from build123d import *

# Parameters (mm, degrees)
SKETCH_W     = 136
SKETCH_H     = 16
SKETCH_R     = 1.65
PAD_DEPTH    = 1
SKETCH001_W  = 106
SKETCH001_H  = 16
PAD001_DEPTH = 3
FILLET_R     = 2


with BuildPart() as part:
    # Sketch → Pad (new body)
    with BuildSketch(Plane.XY):
        Rectangle(SKETCH_W, SKETCH_H)
        with Locations((-60, 4)):
            Circle(SKETCH_R, mode=Mode.SUBTRACT)
        with Locations((-60, -4)):
            Circle(SKETCH_R, mode=Mode.SUBTRACT)
        with Locations((60, 4)):
            Circle(SKETCH_R, mode=Mode.SUBTRACT)
        with Locations((60, -4)):
            Circle(SKETCH_R, mode=Mode.SUBTRACT)
    extrude(amount=PAD_DEPTH)

    # Sketch001 → Pad001 (join)
    with BuildSketch(Plane.XY):
        Rectangle(SKETCH001_W, SKETCH001_H)
    extrude(amount=-PAD001_DEPTH)

    # Fillet
    fillet_edges = [part.edges().sort_by_distance(p)[0] for p in [
        (53, 8, -1.5),
        (53, -8, -1.5),
        (-53, -8, -1.5),
        (-53, 8, -1.5),
        (-68, 8, 0.5),
        (-68, -8, 0.5),
        (68, -8, 0.5),
        (68, 8, 0.5),
    ]]
    fillet(fillet_edges, radius=FILLET_R)


solid = part.part
The model under review builds one solid part; all positions refer to its coordinate system, in mm. A direction names the side the tool comes from. Give positions to 0.01 mm unless a question says otherwise; leave off trailing zeros. Order: outer loops, then holes, each group sorted by start corner. A loop starts at its lowest first (then second) coordinate and runs counter-clockwise, first axis right, second up. Notation, with made-up numbers: M 71,3 L 115,3 A34 cw 115,41 Z; hole C 70,-19 d2. An arc over 180 degrees is marked long. Answer in a Markdown table with one row per item. Add a question column.
1. Machinability: for faces 4 (the flat face through (53, 0, -1)), 5 (the cylindrical face through (-61.65, -3.93, 0.49)), which of the approach directions +Z, -Z, +X, -X, +Y, -Y give a long, thin tool a straight path to every point of the face, cutting with its end or side? Answer none if there is none.
2. To check wall thickness, follow line 1 along Y through (x, z) = (60, 0.85); line 2 along Z through (x, y) = (60.5, -1.5); line 3 along X through (y, z) = (-3, -1.7). State the ranges of each line that lie inside material, in increasing order.
3. Add section A-A on x = 60. State the section outline as (y, z) points.
4. Add section C-C on z = -2.2. State the section outline as (x, y) points, plus the area to 3 significant figures.
5. Add section D-D on y = 1.25. State the section outline as (x, z) points, plus the area to 3 significant figures.
6. Add section B-B on y = -4. State the section outline as (x, z) points, plus the area to 3 significant figures.
7. For pin 1 Ø1.5 at (y, z) = (1, -1) entering from -X; pin 2 Ø2 at (x, y) = (-60, 4) entering from +Z; pin 3 Ø1.5 at (y, z) = (1, -1) entering from +X; pin 4 Ø4.5 at (x, y) = (60, 4) entering from -Z, all flat-tipped, find the tip position at first contact; note any pin that passes through.
8. Mouldability with a two-part tool opening along X and no side actions: class faces 1 (the cylindrical face through (-61.65, 4.07, 0.49)), 2 (the flat face through (-53, 0, -1)), 3 (the flat face through (-1, 8, -1)) as released by +X, released by -X, zero draft, split by the parting line, or undercut.
The answers:
| question | item | result |
|---|---|---|
| 1 | face 4 | -Z, +X, +Y, -Y |
| 1 | face 5 | +Z, -Z |
| 2 | line 1 | -8 to -5.65, -2.35 to 2.35, 5.65 to 8 |
| 2 | line 2 | 0 to 1 |
| 2 | line 3 | -53 to 53 |
| 3 | outline | M -8,0 L -5.65,0 L -5.65,1 L -8,1 Z; M -2.35,0 L 2.35,0 L 2.35,1 L -2.35,1 Z; M 5.65,0 L 8,0 L 8,1 L 5.65,1 Z |
| 4 | outline | M -53,-6 A2 ccw -51,-8 L 51,-8 A2 ccw 53,-6 L 53,6 A2 ccw 51,8 L -51,8 A2 ccw -53,6 Z |
| 4 | area | 1,690 mm2 |
| 5 | outline | M -68,0 L -53,0 L -53,-3 L 53,-3 L 53,0 L 68,0 L 68,1 L -68,1 Z |
| 5 | area | 454 mm2 |
| 6 | outline | M -68,0 L -61.65,0 L -61.65,1 L -68,1 Z; M -58.35,0 L -53,0 L -53,-3 L 53,-3 L 53,0 L 58.35,0 L 58.35,1 L -58.35,1 Z; M 61.65,0 L 68,0 L 68,1 L 61.65,1 Z |
| 6 | area | 447 mm2 |
| 7 | pin 1 | x = -53 |
| 7 | pin 2 | through |
| 7 | pin 3 | x = 53 |
| 7 | pin 4 | z = 0 |
| 8 | face 1 | undercut |
| 8 | face 2 | released by -X |
| 8 | face 3 | zero draft |
